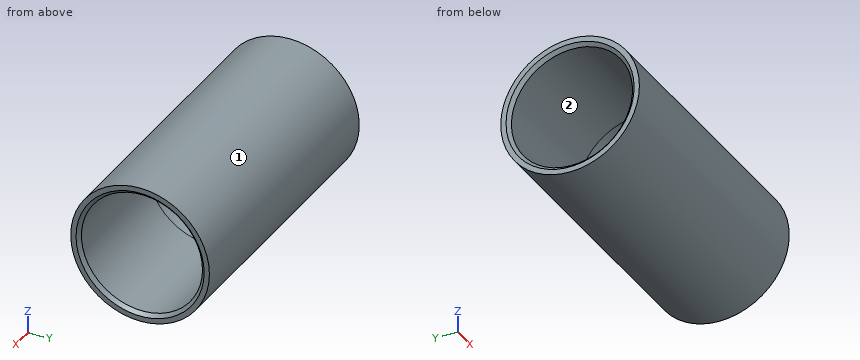
```python
from build123d import *

# Parameters (mm, degrees)
F2_R    = 0.49999
F3_SIZE = 1


# Not quite as in the source:
# - a fillet or chamfer is up to 0.001 mm smaller than in the source, because OpenCascade refuses the exact size


with BuildPart() as f1:
    # F0 (on Top) → F1 (revolve)
    with BuildSketch(Plane.XY):
        Polygon((0, 19.75), (-40, 19.75), (-40, 17.25), (-3.3356409098, 17.25), (-0.5, 16.75), (-0.5, 15.75), (0, 15.75), (0.5, 15.75), (0.5, 16.75), (3.3356409098, 17.25), (40, 17.25), (40, 19.75), align=None)
    revolve(axis=Axis((0, 0, 0), (1, 0, 0)))

    # F2 (radius 0.5 in the source; OpenCascade refuses exactly that, so slightly less here)
    f2_edges = [f1.edges().sort_by_distance(p)[0] for p in [
        (-0.5, -15.75, 0),
        (0.5, -15.75, 0),
    ]]
    fillet(f2_edges, radius=F2_R)

    # F3
    f3_edges = [f1.edges().sort_by_distance(p)[0] for p in [
        (-40, -17.25, 0),
        (40, -17.25, 0),
    ]]
    chamfer(f3_edges, length=F3_SIZE)


solid = f1.part
```
Geometry: final body of the model. Coordinates: model frame, mm. Face numbers are marked on the shaded views. Round coordinates to 2 decimals unless told otherwise and drop trailing zeros. Order: outer loops, then holes, each group sorted by start corner. A loop starts at its lowest first (then second) coordinate and runs counter-clockwise, first axis right, second up. Notation, with made-up numbers: (58, 66) -> (90, 66) arc R17 ccw to (90, 81) -> close; hole circle Ø11 at (36, 81.25). An arc over 180 degrees is marked (long way). Use one line per item in the form item = value. Start each with the question number.
1. Pin query (flat end, axial travel): pin 1 Ø2 at (x, y) = (-27.5, 12) entering from +Z; pin 2 Ø17 at (y, z) = (5.5, -7.5) entering from -X; pin 3 Ø5 at (y, z) = (10, -14) entering from -X; pin 4 Ø6 at (x, y) = (8, 6.5) entering from -Z. Return the tip coordinate at first contact, or that it passes through.
2. Draft query along Y for the marked faces 1 and 2. Return one class per face: pulls with the +Y half, pulls with the -Y half, needs draft (parallel to the pull), parting line crosses it, or undercut.
3. Line query: probe 1 along Z at (x, y) = (0.05, 0); probe 2 along Z at (x, y) = (-29.5, 0); probe 3 along Y at (x, z) = (-19, 5). Output: solid intervals per line, ascending.
4. Cut plane C-C (x = 27.5). Return the cut outline in (y, z).
Solution:
q1.pin_1 = 16.4
q1.pin_2 = -39.55
q1.pin_3 = -40
q1.pin_4 = -19.44
q2.face_1 = parting line crosses it
q2.face_2 = undercut
q3.probe_1 = -19.75 to -15.75, 15.75 to 19.75
q3.probe_2 = -19.75 to -17.25, 17.25 to 19.75
q3.probe_3 = -19.11 to -16.51, 16.51 to 19.11
q4.outline = circle Ø39.5 at (0, 0); hole circle Ø34.5 at (0, 0)
